Read the model definition and answer for the solid it produces. Units are mm, in the model's axes. A direction names the side the tool comes from. Coordinates: 2 decimals unless noted, no trailing zeros. Loops run counter-clockwise (first coordinate to the right, second up) from the corner with the lowest first, then second, coordinate; pieces in that order, holes last. Notation, with made-up numbers: M -3.5,52.5 L 42.5,52.5 A17 cw 42.5,61.5 Z; hole C -15,53.5 d10. An arc over 180 degrees is marked long. One line per item, written item: value. Start each with the question number.
1. The part is cut by section D-D (z = 23). Write down the section's boundary in (x, y), then the cut area to 3 significant figures.
2. The part is cut by section B-B (x = -58.5). Write down the section's boundary in (y, z), then the cut area to 3 significant figures.
3. The part is cut by section A-A (x = -23.5). Write down the section's boundary in (y, z), then the cut area to 3 significant figures.
4. The part is cut by section C-C (z = 40.5). Write down the section's boundary in (x, y).
5. Determine the mould class of faces 4 (the face through (-25, 0, 17)), 5 (the face through (-5, 43, 23)), 6 (the face through (-5, 45, 22)), 7 (the face through (-56.467, 0.986, 23.267)) for opening direction Y: +Y half, -Y half, draft (parallel to the pull), parting line (faces both ways), or undercut.
6. Flat-ended cylindrical pins translate along their axes: pin 1 (3 mm diameter, centred on x = -8, z = 36, fed in from -Y); pin 2 (5 mm diameter, centred on x = -8, z = 10, fed in from -Y); pin 3 (6 mm diameter, centred on y = 14.5, z = 22.5, fed in from -X); pin 4 (1.6 mm diameter, centred on y = 43.5, z = 15.5, fed in from -X). Find the tip coordinate at first contact, or state that the pin passes through.
7. For faces 1 (the face through (-13, 44, 23)), 2 (the face through (-10, 1, 0)), 3 (the face through (-25, 2, 18)), determine the directions among +Z, -Z, +X, -X, +Y, -Y from which every point of the face is accessible in a straight line to the end or side of a thin tool.
8. Consider probe 1 along X at (y, z) = (1.4, 23); probe 2 along Y at (x, z) = (-6, 44); probe 3 along X at (y, z) = (35, 14.5). Determine where each line is inside the solid, lowest interval first.
```python
from build123d import *

# Parameters (mm, degrees)
BOSS_EXTRUDE1_DEPTH = 46
SKETCH2_R           = 13.25
SKETCH2_R_2         = 2.05
CUT_EXTRUDE1_DEPTH  = 2
SKETCH3_R           = 2
CUT_EXTRUDE2_DEPTH  = 100
BOSS_EXTRUDE2_DEPTH = 2


with BuildPart() as part:
    # Sketch1 → Boss-Extrude1 (new body)
    with BuildSketch(Plane.XY):
        Polygon((0, 0), (0, 45), (-13, 45), (-13, 43), (-2, 43), (-2, 2), (-63, 2), (-63, 0), align=None)
    extrude(amount=BOSS_EXTRUDE1_DEPTH)

    # Sketch2 → Cut-Extrude1 (cut)
    with BuildSketch(Plane.XZ):
        with Locations(Location((-41, 23, 0), (0, 0, 270))):
            Circle(SKETCH2_R)
        with Locations(Location((-41, 40.5, 0), (0, 0, 270))):
            Circle(SKETCH2_R_2)
        with Locations(Location((-58.5, 23, 0), (0, 0, 270))):
            Circle(SKETCH2_R_2)
        with Locations(Location((-23.5, 23, 0), (0, 0, 270))):
            Circle(SKETCH2_R_2)
        with Locations(Location((-41, 5.5, 0), (0, 0, 270))):
            Circle(SKETCH2_R_2)
    extrude(amount=-CUT_EXTRUDE1_DEPTH, mode=Mode.SUBTRACT)

    # Sketch3 → Cut-Extrude2 (cut)
    with BuildSketch(Plane(origin=(0, 45, 0), x_dir=(1, 0, 0), z_dir=(0, 1, 0))):
        with Locations(Location((-8, -10, 0), (0, 0, 270))):
            Circle(SKETCH3_R)
        with Locations(Location((-8, -23, 0), (0, 0, 270))):
            Circle(SKETCH3_R)
        with Locations(Location((-8, -36, 0), (0, 0, 270))):
            Circle(SKETCH3_R)
    extrude(amount=-CUT_EXTRUDE2_DEPTH, mode=Mode.SUBTRACT)

    # Sketch4 → Boss-Extrude2 (add)
    with BuildSketch(Plane(origin=(0, 0, 0), x_dir=(-1, 0, 0), z_dir=(0, 0, -1))):
        Polygon((13, 45), (63, 2), (63, 0), (43, 0), (0, 36.98), (0, 45), align=None)
    extrude(amount=BOSS_EXTRUDE2_DEPTH)


solid = part.part
```
Answer block:
1. outline: M -63,0 L -60.55,0 L -60.55,2 L -63,2 Z; M -56.45,0 L -54.25,0 L -54.25,2 L -56.45,2 Z; M -27.75,0 L -25.55,0 L -25.55,2 L -27.75,2 Z; M -21.45,0 L -10,0 L -10,2 L -21.45,2 Z; M -13,43 L -10,43 L -10,45 L -13,45 Z; M -6,0 L 0,0 L 0,45 L -6,45 L -6,43 L -2,43 L -2,2 L -6,2 Z
1. area: 149 mm2
2. outline: M 0,-2 L 5.87,-2 L 5.87,0 L 2,0 L 2,20.95 L 0,20.95 Z; M 0,25.05 L 2,25.05 L 2,46 L 0,46 Z
2. area: 95.5 mm2
3. outline: M 0,0 L 2,0 L 2,20.95 L 0,20.95 Z; M 0,25.05 L 2,25.05 L 2,46 L 0,46 Z; M 16.77,-2 L 35.97,-2 L 35.97,0 L 16.77,0 Z
3. area: 122 mm2
4. outline: M -63,0 L -43.05,0 L -43.05,2 L -63,2 Z; M -38.95,0 L 0,0 L 0,45 L -13,45 L -13,43 L -2,43 L -2,2 L -38.95,2 Z
5. face 4: -Y half
5. face 5: undercut
5. face 6: +Y half
5. face 7: draft
6. pin 1: passes through
6. pin 2: stops at y = 0
6. pin 3: stops at x = -2
6. pin 4: stops at x = -13
7. face 1: +Z, -X, +Y
7. face 2: -Z, +X, -Y
7. face 3: +Z, -X
8. probe 1: x = -63 to -60.55, -56.45 to -54.25, -27.75 to -25.55, -21.45 to -10, -6 to 0
8. probe 2: y = 0 to 2, 43 to 45
8. probe 3: x = -2 to 0
